Verification items for the finished model (mm, model axes). Give positions to 0.01 mm unless a question says otherwise; leave off trailing zeros. Write each loop counter-clockwise with the first axis right and the second up, starting at its lowest first coordinate (ties: lowest second). Pieces come first, ordered by that corner, then holes. Notation, with made-up numbers: M 43.25,-25.5 L 89.25,-25.5 A13 cw 89.25,-7.5 Z; hole C 89,-19 d7. An arc over 180 degrees is marked long. Write item = value, one per line.
from build123d import *

# Parameters (mm, degrees)
F0_W     = 20
F0_H     = 30
F0_H_2   = 5
F0_R     = 1.6
F1_DEPTH = 10.75
F3_DEPTH = 25
F4_W     = 37.611449
F4_H     = 93.224645
F5_DEPTH = 0.1


with BuildPart() as f1:
    # F0 (on Top) → F1 (new body)
    with BuildSketch(Plane.XY):
        Rectangle(F0_W, F0_H)
        with Locations((0, 17.5)):
            Rectangle(F0_W, F0_H_2)
        Polygon((-10, 20), (10, 20), (10, 35.5), (0, 35.5), (-10, 35.5), align=None)
        Polygon((0, 35.5), (10, 35.5), (10, 45.5), (0, 45.5), (-10, 45.5), (-10, 35.5), align=None)
        with Locations((-5, 40.5)):
            Circle(F0_R, mode=Mode.SUBTRACT)
        with Locations((5, 40.5)):
            Circle(F0_R, mode=Mode.SUBTRACT)
    extrude(amount=F1_DEPTH)

    # F2 (on face) → F3 (cut)
    with BuildSketch(Plane.YZ.offset(10)):
        with BuildLine():
            ThreePointArc((20, 10.75), (27.75, 3), (35.5, 10.75))
            Line((35.5, 10.75), (20, 10.75))
        make_face()
        with BuildLine():
            Line((20, 10.75), (35.5, 10.75))
            ThreePointArc((35.5, 10.75), (27.75, 18.5), (20, 10.75))
        make_face()
    extrude(amount=-F3_DEPTH, mode=Mode.SUBTRACT)

    # F4 (on face) → F5 (cut)
    with BuildSketch(Plane.XY.offset(10.75)):
        with Locations((3.746708, 22.084623)):
            Rectangle(F4_W, F4_H)
    extrude(amount=-F5_DEPTH, mode=Mode.SUBTRACT)


solid = f1.part
1) Cross-section at A-A on y = 40.5. Record the boundary of the cut face in (x, z), plus the area to 3 significant figures.
From the geometry:
outline = M -10,0 L -6.6,0 L -6.6,10.65 L -10,10.65 Z; M -3.4,0 L 3.4,0 L 3.4,10.65 L -3.4,10.65 Z; M 6.6,0 L 10,0 L 10,10.65 L 6.6,10.65 Z
area = 145 mm^2
2) Cross-section at B-B on z = 7.25. Record the boundary of the cut face in (x, y).
From the geometry:
outline = M -10,-15 L 10,-15 L 10,20.84 L -10,20.84 Z; M -10,34.66 L 10,34.66 L 10,45.5 L -10,45.5 Z; hole C -5,40.5 d3.2; hole C 5,40.5 d3.2
3) Draft check along Y on faces 1 (the flat face through (0, -15, 5)), 2 (the cylindrical face through (0.1, 27.6, 3)), 3 (the flat face through (10, 15, 5)). Enter one of: +Y half, -Y half, draft (parallel to the pull), parting line (faces both ways), or undercut.
From the geometry:
face_1 = -Y half
face_2 = undercut
face_3 = draft
4) Cross-section at D-D on x = -8.5. Record the boundary of the cut face in (y, z).
From the geometry:
outline = M -15,0 L 45.5,0 L 45.5,10.65 L 35.5,10.65 A7.75 cw 20,10.65 L -15,10.65 Z
5) Material ranges on probe 1 along X at (y, z) = (40.5, 7.25); probe 2 along Y at (x, z) = (5, 4.5); probe 3 along Y at (x, z) = (5, 4.75), recorded low to high. Write a range as from..to.
From the geometry:
probe_1 = -10..-6.6, -3.4..3.4, 6.6..10
probe_2 = -15..23.17, 32.33..38.9, 42.1..45.5
probe_3 = -15..22.84, 32.66..38.9, 42.1..45.5
6) Cross-section at C-C on x = -5. Record the boundary of the cut face in (y, z).
From the geometry:
outline = M -15,0 L 38.9,0 L 38.9,10.65 L 35.5,10.65 A7.75 cw 20,10.65 L -15,10.65 Z; M 42.1,0 L 45.5,0 L 45.5,10.65 L 42.1,10.65 Z
